Build history of the part. All positions in model axes, mm. A direction names the side the tool comes from. Coordinates: 2 decimals unless noted, no trailing zeros. Order: outer loops, then holes, each group sorted by start corner. A loop starts at its lowest first (then second) coordinate and runs counter-clockwise, first axis right, second up. Notation, with made-up numbers: (24.5, 60.25) - (32.5, 60.25) arc R18 ccw to (32.5, 92.25) - close; hole circle Ø9 at (27.5, 58). An arc over 180 degrees is marked (long way). One line per item, written item: value.
from build123d import *

# Parameters (mm, degrees)
SKETCH_1_W          = 70
SKETCH_1_H          = 9
SKETCH_1_R          = 2.1
EXTRUDE_1_DEPTH     = 4.5
SKETCH_3_R          = 4
CUT_EXTRUDE_1_DEPTH = 2.5


with BuildPart() as part:
    # 草圖1 → 填料-伸長1 (new body)
    with BuildSketch(Plane.XY):
        with Locations((15.64232849, -1.657407407)):
            Rectangle(SKETCH_1_W, SKETCH_1_H)
        with Locations((-14.35767151, -1.657407407)):
            Circle(SKETCH_1_R, mode=Mode.SUBTRACT)
        with Locations((15.64232849, -1.657407407)):
            Circle(SKETCH_1_R, mode=Mode.SUBTRACT)
        with Locations((45.64232849, -1.657407407)):
            Circle(SKETCH_1_R, mode=Mode.SUBTRACT)
    extrude(amount=EXTRUDE_1_DEPTH)

    # 草圖3 → 除料-伸長1 (cut)
    with BuildSketch(Plane.XY.offset(4.5)):
        with Locations((-14.35767151, -1.657407407)):
            Circle(SKETCH_3_R)
        with Locations((15.64232849, -1.657407407)):
            Circle(SKETCH_3_R)
        with Locations((45.64232849, -1.657407407)):
            Circle(SKETCH_3_R)
    extrude(amount=-CUT_EXTRUDE_1_DEPTH, mode=Mode.SUBTRACT)


solid = part.part
1. Band-saw the part on A-A, the plane x = -13. Give the cut face in (y, z).
Values found:
outline: (-6.16, 0) - (-3.26, 0) - (-3.26, 2) - (-5.42, 2) - (-5.42, 4.5) - (-6.16, 4.5) - close; (-0.06, 0) - (2.84, 0) - (2.84, 4.5) - (2.11, 4.5) - (2.11, 2) - (-0.06, 2) - close
2. 3-axis set-ups, long thin cutter, end or side, ignore diameter. For faces 1 (the face through (49.46, -0.46, 3.27)), 2 (the face through (15, -6.157, 2)): which of +Z, -Z, +X, -X, +Y, -Y reach the whole face in a straight line?
Values found:
face 1: +Z
face 2: +Z, -Z, +X, -X, -Y
3. Flat gauge pins, fed straight in: P1, Ø4, axis at x = 15.5, y = -2.5, coming from the +Z side; P2, Ø4, axis at x = -14.36, y = -1.66, coming from the +Z side. Where does each tip first touch, or does it go through?
Values found:
P1: stops at z = 2
P2: passes through
4. Band-saw the part on B-B, the plane y = -0.5. Give the cut face in (x, z).
Values found:
outline: (-19.36, 0) - (-16.11, 0) - (-16.11, 2) - (-18.19, 2) - (-18.19, 4.5) - (-19.36, 4.5) - close; (-12.61, 0) - (13.89, 0) - (13.89, 2) - (11.81, 2) - (11.81, 4.5) - (-10.53, 4.5) - (-10.53, 2) - (-12.61, 2) - close; (17.39, 0) - (43.89, 0) - (43.89, 2) - (41.81, 2) - (41.81, 4.5) - (19.47, 4.5) - (19.47, 2) - (17.39, 2) - close; (47.39, 0) - (50.64, 0) - (50.64, 4.5) - (49.47, 4.5) - (49.47, 2) - (47.39, 2) - close
5. Two-plate mould, pull along X, no slides. Class faces 3 (the face through (15, 2.843, 2)), 4 (the face through (-19.358, -2, 2)), 5 (the face through (17.4, -3.4, 2)), 6 (the face through (43.544, -1.565, 0.986)): pulls with the +X half, pulls with the -X half, needs draft (parallel to the pull), parting line crosses it, or undercut.
Values found:
face 3: needs draft
face 4: pulls with the -X half
face 5: undercut
face 6: undercut
6. Band-saw the part on C-C, the plane z = 3.7. Give the cut face in (x, y).
Values found:
outline: (-19.36, -6.16) - (50.64, -6.16) - (50.64, 2.84) - (-19.36, 2.84) - close; hole circle Ø8 at (-14.36, -1.66); hole circle Ø8 at (15.64, -1.66); hole circle Ø8 at (45.64, -1.66)
7. Probe line 1 along X through (y, z) = (-3.5, 3.05); line 2 along X through (y, z) = (-1.75, 0.35); line 3 along Z through (x, y) = (13, -3.75). List the from-to ranges inside material, lowest first.
Values found:
line 1: x = -19.36 to -17.91, -10.81 to 12.09, 19.19 to 42.09, 49.19 to 50.64
line 2: x = -19.36 to -16.46, -12.26 to 13.54, 17.74 to 43.54, 47.74 to 50.64
line 3: z = 0 to 2
